The listing builds one solid part. Answer for the finished solid, in the listing's coordinates (mm). A direction names the side the tool comes from. Round coordinates to 2 decimals unless told otherwise and drop trailing zeros. Loops run counter-clockwise (first coordinate to the right, second up) from the corner with the lowest first, then second, coordinate; pieces in that order, holes last. Notation, with made-up numbers: (60.5, 71) -> (82.5, 71) arc R12 cw to (82.5, 87) -> close; hole circle Ø4 at (29, 85). An arc over 180 degrees is marked (long way). Write each question's results on one line, items separated by ' | '. Start each with the question number.
(1) The part is cut by section D-D (y = -12). Determine the outline of the cut face in (x, z), plus the area to 3 significant figures.
(2) The part is cut by section B-B (z = 4.5). Determine the outline of the cut face in (x, y).
(3) Determine the mould class of faces 4 (the face through (0.53, -4.1, 2.87)), 5 (the face through (-38.1, 37, 18)), 6 (the face through (0.533, -17.633, -5.51)), 7 (the face through (0.53, 19.48, 27.82)) for opening direction Z: released by +Z, released by -Z, zero draft, split by the parting line, or undercut.
(4) The part is cut by section C-C (z = 11). Determine the outline of the cut face in (x, y), plus the area to 3 significant figures.
(5) Straight lines are drawn through the part: probe 1 along Z at (x, y) = (13.5, -6); probe 2 along Z at (x, y) = (31, -7); probe 3 along Y at (x, z) = (-13, 45.5). For each, find the intervals that lie inside material, in ascending order.
(6) The part is cut by section A-A (x = 30). Determine the outline of the cut face in (y, z), plus the area to 3 significant figures.
(7) For faces 1 (the face through (0.53, -5.45, 9.93)), 2 (the face through (38.1, 37, 18)), 3 (the face through (0.53, -3.78, 15.05)), determine the directions among +Z, -Z, +X, -X, +Y, -Y from which every point of the face is accessible in a straight line to the end or side of a thin tool.
(8) Flat-ended cylindrical pins translate along their axes: pin 1 (8 mm diameter, centred on x = -17.5, z = 3.5, fed in from -Y); pin 2 (4 mm diameter, centred on x = -15.5, z = 23.5, fed in from -Y); pin 3 (1 mm diameter, centred on x = 25, y = 24, fed in from +Z); pin 4 (12 mm diameter, centred on y = -8.5, z = 14.5, fed in from -X). Find the tip coordinate at first contact, or state that the pin passes through.
```python
from build123d import *

# Parameters (mm, degrees)
F1_DEPTH = 38.1
F2_R     = 5.08
F3_SIZE  = 5.08


with BuildPart() as f1:
    # F0 (on Right) → F1 (new body, symmetric)
    with BuildSketch(Plane.YZ):
        Polygon((43.706524, 62.419386), (0, 0), (-8.322585, 5.827537), (-2.495048, 14.150121), (-5.095856, 15.971227), (-21.614611, -7.62), (72.976895, -7.62), align=None)
    extrude(amount=F1_DEPTH, both=True)

    # F2
    f2_edges = [f1.edges().sort_by_distance(p)[0] for p in [
        (0, 43.706524, 62.419386),
    ]]
    fillet(f2_edges, radius=F2_R)

    # F3
    f3_edges = [f1.edges().sort_by_distance(p)[0] for p in [
        (0, -21.614611, -7.62),
    ]]
    chamfer(f3_edges, length=F3_SIZE)


solid = f1.part
```
Checked values:
1) outline: (-38.1, -7.62) -> (38.1, -7.62) -> (38.1, 6.11) -> (-38.1, 6.11) -> close | area: 1,050 mm2
2) outline: (-38.1, -13.13) -> (38.1, -13.13) -> (38.1, -6.43) -> (-38.1, -6.43) -> close; (-38.1, 3.15) -> (38.1, 3.15) -> (38.1, 67.91) -> (-38.1, 67.91) -> close
3) face 4: undercut | face 5: zero draft | face 6: released by -Z | face 7: released by +Z
4) outline: (-38.1, -8.58) -> (38.1, -8.58) -> (38.1, -4.7) -> (-38.1, -4.7) -> close; (-38.1, 7.7) -> (38.1, 7.7) -> (38.1, 65.2) -> (-38.1, 65.2) -> close | area: 4,680 mm2
5) probe 1: z = -7.62 to 4.2, 9.14 to 14.68 | probe 2: z = -7.62 to 4.9, 7.72 to 13.25 | probe 3: y = 31.86 to 50.78
6) outline: (-18.7, -3.46) -> (-16.53, -7.62) -> (72.98, -7.62) -> (47.26, 53.91) arc R5.08 ccw to (38.42, 54.86) -> (0, 0) -> (-8.32, 5.83) -> (-2.5, 14.15) -> (-5.1, 15.97) -> close | area: 2,930 mm2
7) face 1: +X, -X | face 2: +Z, -Z, +X, +Y, -Y | face 3: +Z, +X, -X
8) pin 1: stops at y = -16.63 | pin 2: stops at y = 15.05 | pin 3: stops at z = 34.99 | pin 4: stops at x = -38.1
